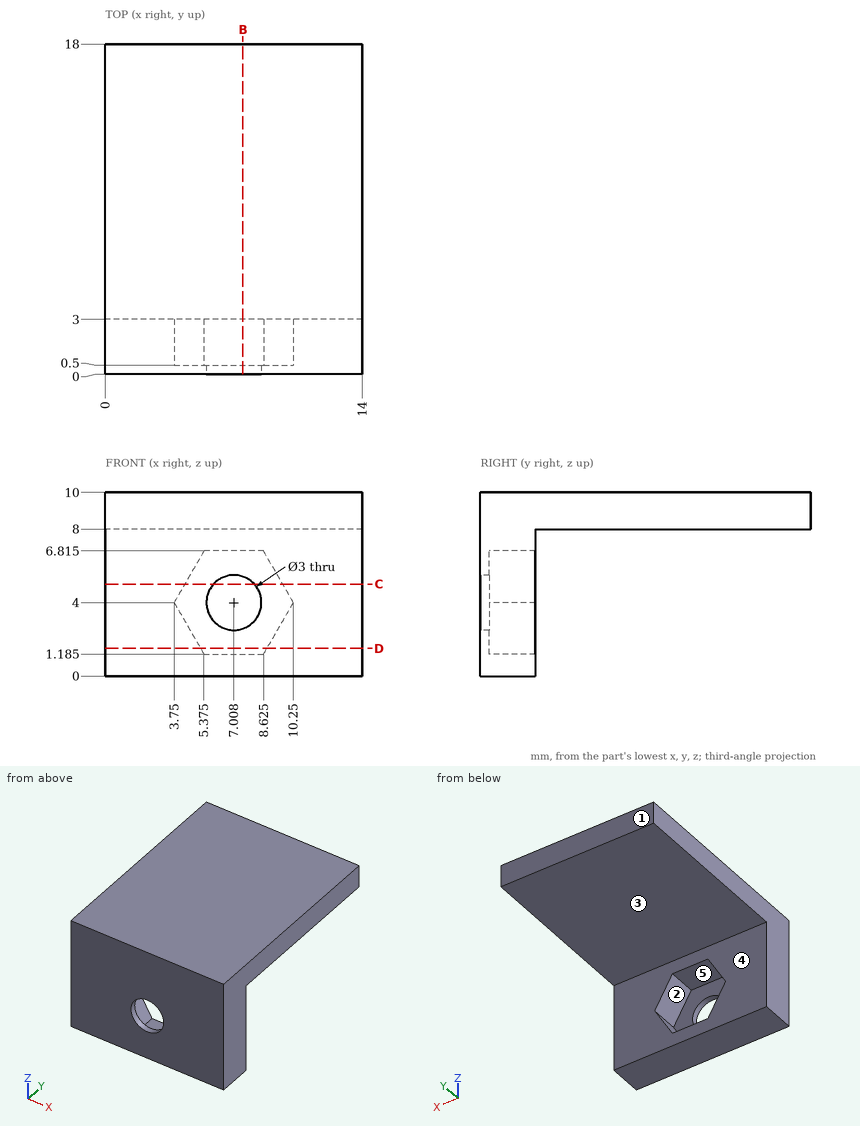
Check sheet for the drawn part. Datum: minimum x, y, z corner. Units: mm. A direction names the side the tool comes from. Give positions to 0.01 mm unless a question says otherwise; leave off trailing zeros. Write each loop counter-clockwise with the first axis right and the second up, starting at its lowest first coordinate (ties: lowest second). Pieces come first, ordered by that corner, then holes. Notation, with made-up numbers: M 5.5,87.5 L 51.5,87.5 A19 cw 51.5,113.5 Z; hole C 31,-10 d5. An arc over 180 degrees is marked long. One line per question, with ' | ' between items.
1) Set-up check for the marked faces 1 and 2: record each of +Z, -Z, +X, -X, +Y, -Y from which the full face is reachable in a straight line by a thin tool's end or side.
Result:
face 1: +Z, -Z, +X, -X, +Y | face 2: +Y
2) Section check C-C on z = 5. Enter the section's corners in (x, y).
Result:
outline: M 0,0 L 5.89,0 L 5.89,0.5 L 4.33,0.5 L 4.33,3 L 0,3 Z; M 8.13,0 L 14,0 L 14,3 L 9.67,3 L 9.67,0.5 L 8.13,0.5 Z
3) Mould release check, pull along Z, two halves, no side actions. Record for the marked faces 3, 4 and 5: released by +Z, released by -Z, zero draft, split by the parting line, or undercut.
Result:
face 3: released by -Z | face 4: zero draft | face 5: undercut
4) Thickness scan on line 1 along Y through (x, z) = (3.5, 0.5); line 2 along Z through (x, y) = (8.25, 1.75) (1 decimal); line 3 along Z through (x, y) = (11, 11.25). Record the ranges inside material, lowest first. Write a range as [from, to].
Result:
line 1: y = [0, 3] | line 2: z = [0, 1.2], [6.8, 10] | line 3: z = [8, 10]
5) Section check D-D on z = 1.5. Enter the section's corners in (x, y).
Result:
outline: M 0,0 L 14,0 L 14,3 L 8.81,3 L 8.81,0.5 L 5.19,0.5 L 5.19,3 L 0,3 Z
6) Section check B-B on x = 7.5. Enter the section's corners in (y, z) (1 decimal).
Result:
outline: M 0,0 L 3,0 L 3,1.2 L 0.5,1.2 L 0.5,2.6 L 0,2.6 Z; M 0,5.4 L 0.5,5.4 L 0.5,6.8 L 3,6.8 L 3,8 L 18,8 L 18,10 L 0,10 Z
7) Gauge pin test, flat ends, axial feed: pin 1 Ø7 at (x, y) = (9.5, 8.5) entering from -Z; pin 2 Ø6 at (x, z) = (7.5, 4) entering from +Y; pin 3 Ø2.5 at (x, z) = (7.5, 5.5) entering from +Y. Record the tip position at first contact, or that the pin passes through.
Result:
pin 1: stops at z = 8 | pin 2: stops at y = 3 | pin 3: stops at y = 0.5
